Check sheet for the modelled part. Datum: model origin and axes. Units: mm. A direction names the side the tool comes from. Give positions to 0.01 mm unless a question says otherwise; leave off trailing zeros. Loops run counter-clockwise (first coordinate to the right, second up) from the corner with the lowest first, then second, coordinate; pieces in that order, holes last. Notation, with made-up numbers: M -10.5,-15.5 L 9.5,-15.5 A29 ccw 9.5,4.5 Z; hole C 5.25,45.5 d1. An arc over 180 degrees is marked long. Use one line per item in the form item = value.
from build123d import *

# Parameters (mm, degrees)
BOSS_EXTRUDE1_DEPTH = 52
BOSS_EXTRUDE2_DEPTH = 4


with BuildPart() as part:
    # Sketch1 → Boss-Extrude1 (new body)
    with BuildSketch(Plane.XY):
        with BuildLine():
            Line((-37.913907285, 9), (-37.913907285, 0))
            Line((-37.913907285, 0), (37.086092715, 0))
            Line((37.086092715, 0), (37.086092715, 9))
            Line((37.086092715, 9), (4.086092715, 9))
            Line((4.086092715, 9), (4.086092715, 24.793471725))
            ThreePointArc((4.086092715, 24.793471725), (18.520210619, 33.261347251), (24.207343925, 49))
            Line((24.207343925, 49), (16.207343925, 49))
            ThreePointArc((16.207343925, 49), (-0.413907285, 32.37874879), (-17.035158495, 49))
            Line((-17.035158495, 49), (-25.035158495, 49))
            ThreePointArc((-25.035158495, 49), (-19.348025189, 33.261347251), (-4.913907285, 24.793471725))
            Line((-4.913907285, 24.793471725), (-4.913907285, 9))
            Line((-4.913907285, 9), (-37.913907285, 9))
        make_face()
    extrude(amount=-BOSS_EXTRUDE1_DEPTH)


with BuildPart() as part_1:
    # Body-Move/Copy1: moved
    add(part.part.moved(Location((0, 0, 26))))

    # Sketch3 → Boss-Extrude2 (add, symmetric)
    with BuildSketch(Plane.XY):
        with BuildLine():
            Line((24.207343925, 49), (37.086092715, 9))
            Line((37.086092715, 9), (4.086092715, 9))
            Line((4.086092715, 9), (4.086092715, 24.793471725))
            ThreePointArc((4.086092715, 24.793471725), (18.520210619, 33.261347251), (24.207343925, 49))
        make_face()
        with BuildLine():
            Line((-25.035158495, 49), (-37.913907285, 9))
            Line((-37.913907285, 9), (-4.913907285, 9))
            Line((-4.913907285, 9), (-4.913907285, 24.793471725))
            ThreePointArc((-4.913907285, 24.793471725), (-19.348025189, 33.261347251), (-25.035158495, 49))
        make_face()
    extrude(amount=BOSS_EXTRUDE2_DEPTH, both=True)


solid = part_1.part
1) Set-up check for faces 1 (the face through (-1, 19, -26)), 2 (the face through (-19.5, 33.446, -14.846)), 3 (the face through (21, 9, -15)), 4 (the face through (-19.5, 33.446, 15.154)), 5 (the face through (18.37, 33.08, 15.15)): record each of +Z, -Z, +X, -X, +Y, -Y from which the full face is reachable in a straight line by a thin tool's end or side.
Evaluation:
face_1 = -Z, +X, -X, +Y, -Y
face_2 = -Z, -X
face_3 = -Z, +X
face_4 = +Z, -X
face_5 = +Z, +X
2) Section check D-D (y = 40). Record the cut outline in (x, z).
Evaluation:
outline = M -27.93,-4 L -23.33,-4 L -23.33,-26 L -14.39,-26 L -14.39,26 L -23.33,26 L -23.33,4 L -27.93,4 Z; M 13.56,-26 L 22.5,-26 L 22.5,-4 L 27.11,-4 L 27.11,4 L 22.5,4 L 22.5,26 L 13.56,26 Z
3) Scan lines: line 1 (Z direction, x = 4.5, y = 13); line 2 (X direction, y = 42, z = -2); line 3 (X direction, y = 19, z = -16.5). Record each from-to range of solid material in increasing order.
Evaluation:
line_1 = -4 to 4
line_2 = -27.29 to -15.49, 14.66 to 26.46
line_3 = -4.91 to 4.09
4) Release check for a two-part mould opening along X. For faces 6 (the face through (-0.048, 32.383, 0.364)), 7 (the face through (18.37, 33.08, -14.85)), 8 (the face through (-31.384, 29.28, 0.056)), 9 (the face through (21, 20, -4)) record: pulls with the +X half, pulls with the -X half, needs draft (parallel to the pull), parting line crosses it, or undercut.
Evaluation:
face_6 = undercut
face_7 = pulls with the +X half
face_8 = pulls with the -X half
face_9 = needs draft
5) Section check B-B (x = 6). Record the cut outline in (y, z).
Evaluation:
outline = M 0,-26 L 9,-26 L 9,-4 L 25.23,-4 L 25.23,-26 L 33.67,-26 L 33.67,26 L 25.23,26 L 25.23,4 L 9,4 L 9,26 L 0,26 Z
6) Depth check by flat-ended pin: pin 1 Ø10 at (x, z) = (2.5, 4.5) entering from +Y; pin 2 Ø5 at (x, y) = (-29, 26.5) entering from -Z; pin 3 Ø16.5 at (x, y) = (25, 20) entering from +Z. Enter the tip coordinate at first touch or a pass-through.
Evaluation:
pin_1 = 34.38
pin_2 = -4
pin_3 = 4
7) Section check C-C (z = -6). Record the cut outline in (x, y).
Evaluation:
outline = M -37.91,0 L 37.09,0 L 37.09,9 L 4.09,9 L 4.09,24.79 A24.62 ccw 24.21,49 L 16.21,49 A16.62 cw -17.04,49 L -25.04,49 A24.62 ccw -4.91,24.79 L -4.91,9 L -37.91,9 Z
8) Section check A-A (y = 34). Record the cut outline in (x, z).
Evaluation:
outline = M -29.86,-4 L -19.94,-4 L -19.94,-26 L -7.57,-26 L -7.57,26 L -19.94,26 L -19.94,4 L -29.86,4 Z; M 6.75,-26 L 19.11,-26 L 19.11,-4 L 29.04,-4 L 29.04,4 L 19.11,4 L 19.11,26 L 6.75,26 Z
